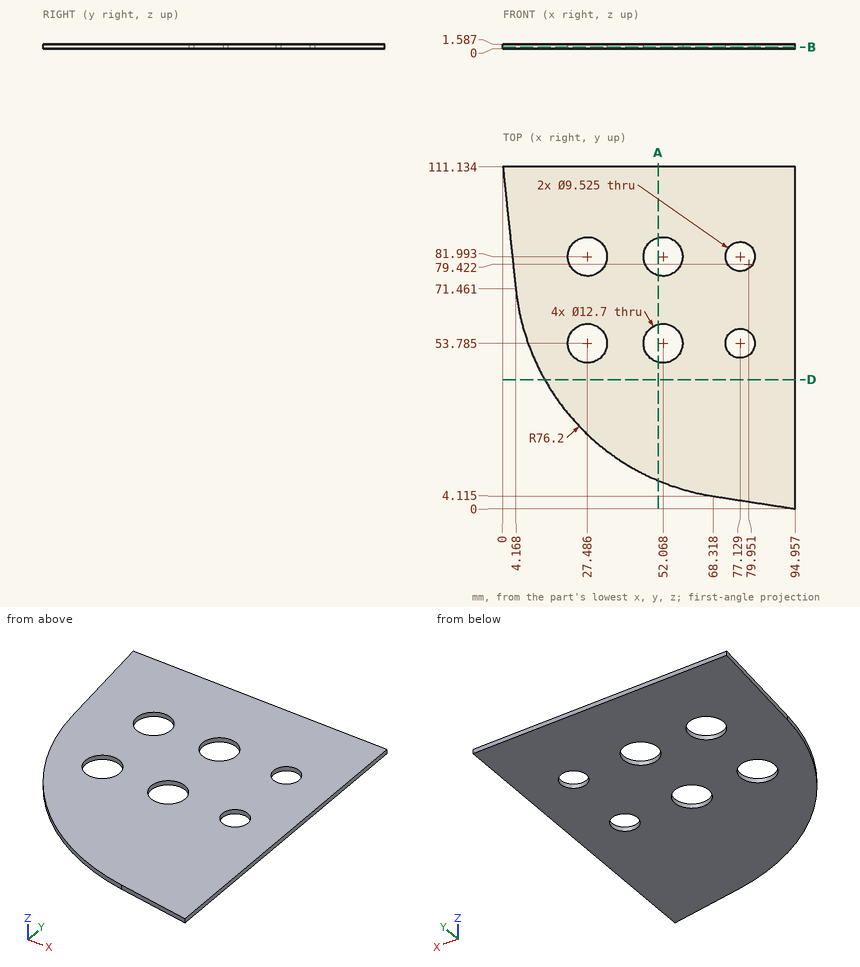
For this review, use the dimensioned drawing (mm, ordinates from the lowest corner) and the shaded views. Round coordinates to 2 decimals unless told otherwise and drop trailing zeros. Loops run counter-clockwise (first coordinate to the right, second up) from the corner with the lowest first, then second, coordinate; pieces in that order, holes last. Notation, with made-up numbers: M -5,-18.75 L 3,-18.75 A13 ccw 3,6.25 Z; hole C 82,51 d7. An arc over 180 degrees is marked long. Answer as a JSON object with one key per item and string values.
(1) Take a section at A-A on x = 50.5. Give the boundary of the cut face in (y, z) (1 decimal), and give its area (3 significant figures).
Resolved:
{"outline": "M 9.1,0 L 47.6,0 L 47.6,1.6 L 9.1,1.6 Z; M 59.9,0 L 75.8,0 L 75.8,1.6 L 59.9,1.6 Z; M 88.1,0 L 111.1,0 L 111.1,1.6 L 88.1,1.6 Z", "area": "123 mm²"}
(2) To check wall thickness, follow line 1 along Y through (x, z) = (31.5, 1) (1 decimal); line 2 along X through (y, z) = (86, 0.15) (1 decimal); line 3 along Y through (x, z) = (37, 0.35) (1 decimal). State the ranges of each line that lie inside material, in increasing order.
Resolved:
{"line 1": "20.6 to 48.9, 58.7 to 77.1, 86.9 to 111.1", "line 2": "2.6 to 22.6, 32.4 to 47.1, 57 to 74.6, 79.7 to 95", "line 3": "16.5 to 111.1"}
(3) Take a section at B-B on z = 0.55. Count the separate pieces of the cut face and the enclosed holes in it, and give its area (3 significant figures).
Resolved:
{"separate pieces": "1", "enclosed holes": "6", "area": "8,050 mm²"}
(4) Clearance check with flat-ended pins moving along their axes: P1, Ø7.5, axis at x = 52.07, y = 81.99, coming from the +Z side; P2, Ø16.5, axis at x = 27.49, y = 53.79, coming from the -Z side. State where each tip first meets the part, or that it passes through.
Resolved:
{"P1": "through", "P2": "z = 0"}
(5) Take a section at D-D on y = 42. Give the boundary of the cut face in (x, z), and give its area (3 significant figures).
Resolved:
{"outline": "M 13.57,0 L 94.96,0 L 94.96,1.59 L 13.57,1.59 Z", "area": "129 mm²"}
